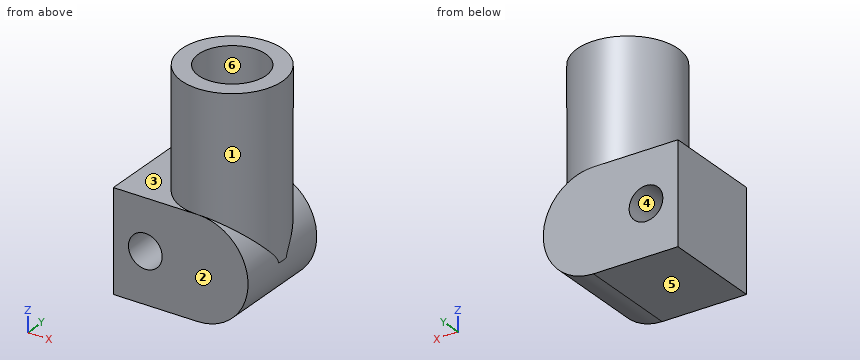
from build123d import *

# Parameters (mm, degrees)
SKETCH1_R           = 7.5
SKETCH1_R_2         = 5
BOSS_EXTRUDE1_DEPTH = 25
BOSS_EXTRUDE3_DEPTH = 7.5
SKETCH5_R           = 2.5
CUT_EXTRUDE3_DEPTH  = 15


with BuildPart() as part:
    # Sketch1 → Boss-Extrude1 (new body)
    with BuildSketch(Plane.XY):
        Circle(SKETCH1_R)
        Circle(SKETCH1_R_2, mode=Mode.SUBTRACT)
    extrude(amount=BOSS_EXTRUDE1_DEPTH)

    # Sketch4 → Boss-Extrude3 (add, symmetric)
    with BuildSketch(Plane(origin=(0, 0, 0), x_dir=(1, 0, 0), z_dir=(0, 1, 0))):
        with BuildLine():
            Line((0, -7.449392631), (-9.305010791, -7.449392631))
            Line((-9.305010791, -7.449392631), (-12.541569439, -7.449392631))
            Line((-12.541569439, -7.449392631), (-12.541569439, 7.449392631))
            Line((-12.541569439, 7.449392631), (-9.305010791, 7.449392631))
            Line((-9.305010791, 7.449392631), (0, 7.449392631))
            ThreePointArc((0, 7.449392631), (7.449392631, 0), (0, -7.449392631))
        make_face()
    extrude(amount=BOSS_EXTRUDE3_DEPTH, both=True)

    # Sketch5 → Cut-Extrude3 (cut)
    with BuildSketch(Plane(origin=(0, 7.5, 0), x_dir=(1, 0, 0), z_dir=(0, 1, 0))):
        with Locations(Location((-7.8, 0, 0), (0, 0, 270))):
            Circle(SKETCH5_R)
    extrude(amount=-CUT_EXTRUDE3_DEPTH, mode=Mode.SUBTRACT)


solid = part.part
Input: part model. Units: mm. Frame: model coordinates. Face numbers are marked on the shaded views. A direction names the side the tool comes from. Coordinates: 2 decimals unless noted, no trailing zeros. Loops run counter-clockwise (first coordinate to the right, second up) from the corner with the lowest first, then second, coordinate; pieces in that order, holes last. Notation, with made-up numbers: (-4.5, 7) -> (50.5, 7) arc R12 cw to (50.5, 21) -> close; hole circle Ø4 at (13.5, 75.25). An arc over 180 degrees is marked (long way). Write item = value, one per line. Start each with the question number.
Item 1: First-contact query: P1, Ø6, axis at x = -6.5, z = 1.5, coming from the -Y side; P2, Ø4, axis at x = -7.8, z = 0, coming from the -Y side; P3, Ø3, axis at x = 5, z = 20, coming from the +Y side; P4, Ø4, axis at y = 2.5, z = 6.5, coming from the +X side. Flat tips, straight axial feed; report the tip coordinate or a pass-through.
Item 2: Cut plane A-A, the plane y = 0. Return loops of the section in (x, z), plus the area to 3 significant figures.
Item 3: Cut plane B-B, the plane x = -6. Return loops of the section in (y, z), plus the area to 3 significant figures.
Item 4: Reachability of the marked faces 1 and 2 from +Z, -Z, +X, -X, +Y, -Y: full face, straight path, thin tool, end or side. Return the list, or none.
Item 5: Mould query, pull axis Z, two halves, no side actions, for the marked faces 3, 4, 5 and 6. Classes: pulls with the +Z half, pulls with the -Z half, needs draft (parallel to the pull), parting line crosses it, or undercut.
Item 6: Material intervals for line 1 (Y direction, x = 0, z = 18); line 2 (X direction, y = 2, z = 0), sorted ascending.
Item 7: Cut plane C-C, the plane z = -1. Return loops of the section in (x, y).
Item 8: Cut plane D-D, the plane z = 11. Return loops of the section in (x, y).
Ans:
q1.P1 = -7.5
q1.P2 = through
q1.P3 = 6.63
q1.P4 = 7.48
q2.outline = (-12.54, -7.45) -> (0, -7.45) arc R7.45 ccw to (7.45, 0) -> (7.5, 0) -> (7.5, 25) -> (5, 25) -> (5, 5.52) arc R7.45 ccw to (0, 7.45) -> (-5, 7.45) -> (-5, 25) -> (-7.5, 25) -> (-7.5, 7.45) -> (-12.54, 7.45) -> close; hole circle Ø5 at (-7.8, 0)
q2.area = 351 mm²
q3.outline = (-7.5, -7.45) -> (7.5, -7.45) -> (7.5, -1.73) -> (-7.5, -1.73) -> close; (-7.5, 1.73) -> (7.5, 1.73) -> (7.5, 7.45) -> (4.5, 7.45) -> (4.5, 25) -> (-4.5, 25) -> (-4.5, 7.45) -> (-7.5, 7.45) -> close
q3.area = 329 mm²
q4.face_1 = +Z
q4.face_2 = +Z, -Z, +X, -X, -Y
q5.face_3 = pulls with the +Z half
q5.face_4 = undercut
q5.face_5 = pulls with the -Z half
q5.face_6 = needs draft
q6.line_1 = -7.5 to -5, 5 to 7.5
q6.line_2 = -12.54 to -10.3, -5.3 to 7.45
q7.outline = (-12.54, -7.5) -> (-10.09, -7.5) -> (-10.09, 7.5) -> (-12.54, 7.5) -> close; (-5.51, -7.5) -> (7.38, -7.5) -> (7.38, 7.5) -> (-5.51, 7.5) -> close
q8.outline = circle Ø15 at (0, 0); hole circle Ø10 at (0, 0)
